The model under review builds one solid part; all positions refer to its coordinate system, in mm. A direction names the side the tool comes from. Coordinates: 2 decimals unless noted, no trailing zeros. Order: outer loops, then holes, each group sorted by start corner. A loop starts at its lowest first (then second) coordinate and runs counter-clockwise, first axis right, second up. Notation, with made-up numbers: (2.25, -4.5) -> (53.25, -4.5) arc R29 cw to (53.25, 26.5) -> close; hole circle Ø9 at (-8.5, -7.75). An arc over 180 degrees is marked (long way). Use one line per item in the form item = value. Start each with the question number.
(1) Wall thickness on line 1 along Y through (x, z) = (1196, 37); line 2 along X through (y, z) = (188, 32.5); line 3 along Z through (x, y) = (164, 134.5): over which ranges is each line inside the solid? List them lowest first.
(2) For faces 4 (the flat face through (1953.26, 502, 29)), 5 (the flat face through (964, 502, 0)), list the 3-axis set-ups (+Z, -Z, +X, -X, +Y, -Y) from which the entire face can be reached by the end or side of a thin tool; tool diameter is ignored.
(3) Take a section at C-C (x = 496). State the section outline as (y, z) points.
(4) Insertion check: pin 1 Ø3 at (x, y) = (969.5, 269.5) entering from +Z. The pin has a flat end and moves straight along its axis. Give the tip position at first contact, or say it passes through.
(5) Mouldability with a two-part tool opening along Y and no side actions: class faces 1 (the flat face through (964, 0, 24)), 2 (the flat face through (964, 502, 10.16)), 3 (the flat face through (1955.8, 488, 24)) as +Y half, -Y half, draft (parallel to the pull), parting line (faces both ways), or undercut.
(6) Take a section at B-B (y = 437). State the section outline as (x, z) points.
(7) Take a section at A-A (z = 36). State the section outline as (x, y) points, then the cut area to 3 significant figures.
```python
from build123d import *

# Parameters (mm, degrees)
F0_W     = 1955.8
F0_H     = 990.6
F1_DEPTH = 10.16
F3_DEPTH = 38.1


with BuildPart() as f1:
    # F0 (on Top) → F1 (new body)
    with BuildSketch(Plane.XY):
        with Locations((977.9, 495.3)):
            Rectangle(F0_W, F0_H)
    extrude(amount=F1_DEPTH)

    # F2 (on face) → F3 (join)
    with BuildSketch(Plane.XY.offset(10.16)):
        Polygon((2.54, 125.157505), (0, 125.157505), (0, 0), (9.51278, 0), (9.51278, 2.54), (2.54, 2.54), align=None)
        Polygon((0, 990.6), (0, 125.157505), (2.54, 125.157505), (2.54, 988.06), (1948.808074, 988.06), (1948.808074, 990.6), align=None)
        Polygon((1955.8, 990.6), (1948.808074, 990.6), (1948.808074, 988.06), (1953.26, 988.06), (1953.26, 977.438092), (1955.8, 977.438092), align=None)
        Polygon((9.51278, 2.54), (9.51278, 0), (1955.8, 0), (1955.8, 977.438092), (1953.26, 977.438092), (1953.26, 2.54), align=None)
    extrude(amount=F3_DEPTH)


solid = f1.part
```
Findings:
q1.line_1 = 0 to 2.54, 988.06 to 990.6
q1.line_2 = 0 to 2.54, 1953.26 to 1955.8
q1.line_3 = 0 to 10.16
q2.face_4 = +Z
q2.face_5 = -Z, +X, -X, +Y, -Y
q3.outline = (0, 0) -> (990.6, 0) -> (990.6, 48.26) -> (988.06, 48.26) -> (988.06, 10.16) -> (2.54, 10.16) -> (2.54, 48.26) -> (0, 48.26) -> close
q4.pin_1 = 10.16
q5.face_1 = -Y half
q5.face_2 = undercut
q5.face_3 = draft
q6.outline = (0, 0) -> (1955.8, 0) -> (1955.8, 48.26) -> (1953.26, 48.26) -> (1953.26, 10.16) -> (2.54, 10.16) -> (2.54, 48.26) -> (0, 48.26) -> close
q7.outline = (0, 0) -> (1955.8, 0) -> (1955.8, 990.6) -> (0, 990.6) -> close; hole (2.54, 2.54) -> (1953.26, 2.54) -> (1953.26, 988.06) -> (2.54, 988.06) -> close
q7.area = 14,900 mm²
